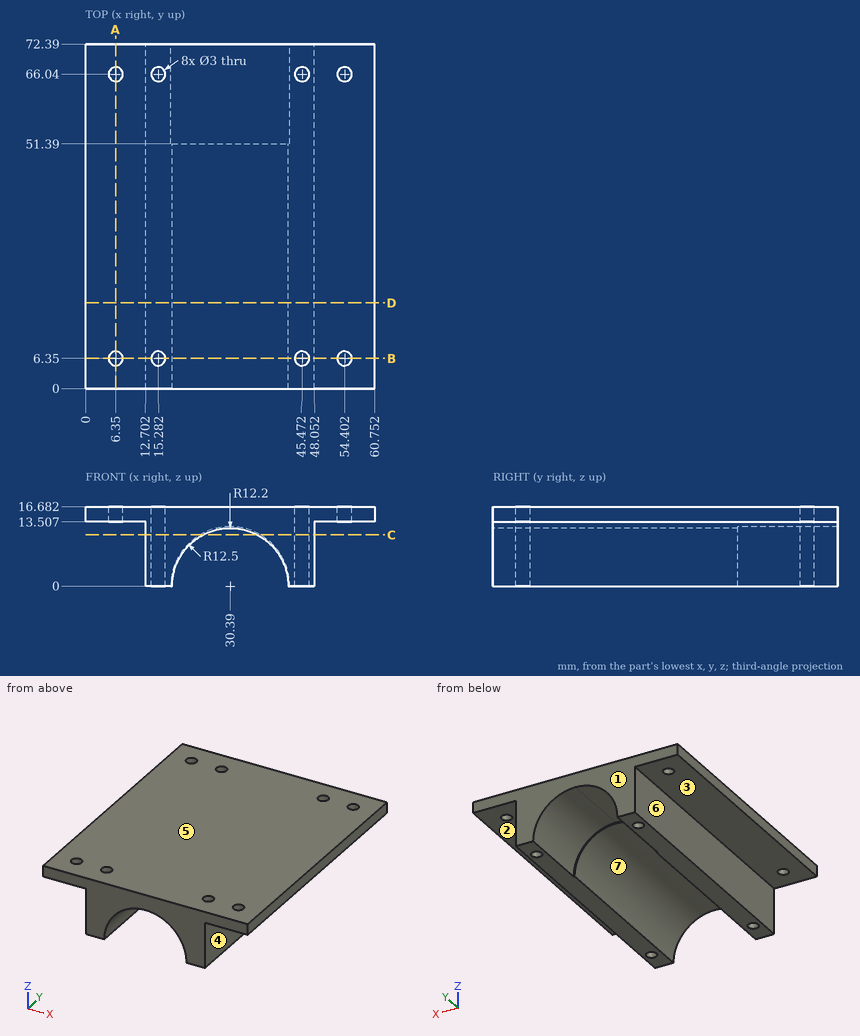
For this review, use the dimensioned drawing (mm, ordinates from the lowest corner) and the shaded views. A direction names the side the tool comes from. Round coordinates to 2 decimals unless told otherwise and drop trailing zeros. Write each loop counter-clockwise with the first axis right and the second up, starting at its lowest first coordinate (ties: lowest second). Pieces come first, ordered by that corner, then holes. Notation, with made-up numbers: (33, 72.5) - (53, 72.5) arc R23 cw to (53, 105.5) - close; hole circle Ø4 at (53, 15). An arc over 180 degrees is marked (long way). Answer as CSV lines item,"result". Start each with the question number.
(1) We need section B-B on y = 6.35. State the section outline as (x, z) points.
(2) Draft analysis for pull direction X (two halves, no side actions). For the marked faces 4, 5, 6 and 7, state which applies: pulls with the +X half, pulls with the -X half, needs draft (parallel to the pull), parting line crosses it, or undercut.
(3) We need section D-D on y = 18. State the section outline as (x, z) points.
(4) We need section A-A on x = 6.35. State the section outline as (y, z) points, plus the area to 3 significant figures.
(5) We need section C-C on z = 10.75. State the section outline as (x, y) points.
(6) For pin 1 Ø7 at (y, z) = (46, 9.5) entering from +X; pin 2 Ø6.5 at (x, y) = (8.5, 21.5) entering from -Z; pin 3 Ø5 at (x, z) = (51, 10) entering from -Y, all flat-tipped, find the tip position at first contact; note any pin that passes through.
(7) For the marked faces 1, 2 and 3, list the 3-axis set-ups (+Z, -Z, +X, -X, +Y, -Y) from which the entire face can be reached by the end or side of a thin tool; tool diameter is ignored.
(8) To check wall thickness, follow line 1 (X direction, y = 66.04, z = 15.15); line 2 (X direction, y = 49, z = 8.5); line 3 (Z direction, x = 58.5, y = 17). State the ranges of each line that lie inside material, in increasing order.
Worked answers:
1,outline,"(0, 13.51) - (4.85, 13.51) - (4.85, 16.68) - (0, 16.68) - close; (7.85, 13.51) - (12.7, 13.51) - (12.7, 0) - (13.78, 0) - (13.78, 16.68) - (7.85, 16.68) - close; (16.78, 0) - (18.19, 0) arc R12.2 cw to (42.59, 0) - (43.97, 0) - (43.97, 16.68) - (16.78, 16.68) - close; (46.97, 0) - (48.05, 0) - (48.05, 13.51) - (52.9, 13.51) - (52.9, 16.68) - (46.97, 16.68) - close; (55.9, 13.51) - (60.75, 13.51) - (60.75, 16.68) - (55.9, 16.68) - close"
2,face 4,"pulls with the +X half"
2,face 5,"needs draft"
2,face 6,"pulls with the -X half"
2,face 7,"undercut"
3,outline,"(0, 13.51) - (12.7, 13.51) - (12.7, 0) - (18.19, 0) arc R12.2 cw to (42.59, 0) - (48.05, 0) - (48.05, 13.51) - (60.75, 13.51) - (60.75, 16.68) - (0, 16.68) - close"
4,outline,"(0, 13.51) - (4.85, 13.51) - (4.85, 16.68) - (0, 16.68) - close; (7.85, 13.51) - (64.54, 13.51) - (64.54, 16.68) - (7.85, 16.68) - close; (67.54, 13.51) - (72.39, 13.51) - (72.39, 16.68) - (67.54, 16.68) - close"
4,area,"211 mm²"
5,outline,"(12.7, 0) - (24.62, 0) - (24.62, 51.39) - (24.01, 51.39) - (24.01, 72.39) - (12.7, 72.39) - close; (36.16, 0) - (48.05, 0) - (48.05, 72.39) - (36.77, 72.39) - (36.77, 51.39) - (36.16, 51.39) - close; hole circle Ø3 at (15.28, 6.35); hole circle Ø3 at (15.28, 66.04); hole circle Ø3 at (45.47, 6.35); hole circle Ø3 at (45.47, 66.04)"
6,pin 1,"x = 48.05"
6,pin 2,"z = 13.51"
6,pin 3,"through"
7,face 1,"+Z, -Z, +X, -X, +Y"
7,face 2,"-Z, +X, +Y, -Y"
7,face 3,"-Z, -X, +Y, -Y"
8,line 1,"0 to 4.85, 7.85 to 13.78, 16.78 to 43.97, 46.97 to 52.9, 55.9 to 60.75"
8,line 2,"12.7 to 21.64, 39.14 to 48.05"
8,line 3,"13.51 to 16.68"
